Read the model definition and answer for the solid it produces. Units are mm, in the model's axes. A direction names the side the tool comes from. Round coordinates to 2 decimals unless told otherwise and drop trailing zeros. Write each loop counter-clockwise with the first axis right and the second up, starting at its lowest first coordinate (ties: lowest second). Pieces come first, ordered by that corner, then holes.
from build123d import *

# Parameters (mm, degrees)
BOSS_EXTRUDE1_DEPTH = 6.35
SKETCH2_R           = 5.08
BOSS_EXTRUDE2_DEPTH = 6.35
SKETCH3_R           = 5.08
BOSS_EXTRUDE3_DEPTH = 19.05
SKETCH4_R           = 3.81
CUT_EXTRUDE1_DEPTH  = 32.75
CUT_EXTRUDE2_DEPTH  = 15.24
CIRPATTERN1_COUNT   = 6


with BuildPart() as part:
    # Sketch1 → Boss-Extrude1 (new body)
    with BuildSketch(Plane.XY):
        Polygon((0, 8.248891971), (-7.14375, 4.124445986), (-7.14375, -4.124445986), (0, -8.248891971), (7.14375, -4.124445986), (7.14375, 4.124445986), align=None)
    extrude(amount=BOSS_EXTRUDE1_DEPTH)

    # Sketch2 → Boss-Extrude2 (add)
    with BuildSketch(Plane(origin=(0, 0, 0), x_dir=(-1, 0, 0), z_dir=(0, 0, -1))):
        Circle(SKETCH2_R)
    extrude(amount=BOSS_EXTRUDE2_DEPTH)

    # Sketch3 → Boss-Extrude3 (add)
    with BuildSketch(Plane.XY.offset(6.35)):
        Circle(SKETCH3_R)
    extrude(amount=BOSS_EXTRUDE3_DEPTH)

    # Sketch4 → Cut-Extrude1 (cut, through all)
    with BuildSketch(Plane.XY.offset(25.4)):
        Circle(SKETCH4_R)
    extrude(amount=-CUT_EXTRUDE1_DEPTH, mode=Mode.SUBTRACT)

    # Sketch5 → Cut-Extrude2 (cut)
    with BuildSketch(Plane.XY.offset(25.4)):
        Polygon((0, 4.810914796), (0.765045953, 4.810914796), (1.27, 5.114868927), (0, 5.114868927), (-1.27, 5.114868927), (-0.765045953, 4.810914796), align=None)
    cut_extrude2 = extrude(amount=-CUT_EXTRUDE2_DEPTH, mode=Mode.SUBTRACT)

    # CirPattern1: Cut-Extrude2 ×6 about axis
    cirpattern1_axis = Axis((0, 0, 0), (0, 0, 1))
    for i in range(1, CIRPATTERN1_COUNT):
        add(cut_extrude2.rotate(cirpattern1_axis, i * 360 / CIRPATTERN1_COUNT), mode=Mode.SUBTRACT)


solid = part.part
Q1. Determine the mould class of faces 1 (the cylindrical face through (-0.83, -3.72, 9.75)), 2 (the flat face through (3.522, -6.216, 3.131)), 3 (the flat face through (-3.522, 6.216, 3.131)) for opening direction X: pulls with the +X half, pulls with the -X half, needs draft (parallel to the pull), parting line crosses it, or undercut.
Verdict:
face 1: undercut
face 2: pulls with the +X half
face 3: pulls with the -X half
Q2. Straight lines are drawn through the part: probe 1 along Y at (x, z) = (0, 13); probe 2 along Y at (x, z) = (0, 8.5); probe 3 along Z at (x, y) = (4, 4.5). For each, find the intervals that lie inside material, in ascending order.
Verdict:
probe 1: y = -4.81 to -3.81, 3.81 to 4.81
probe 2: y = -5.08 to -3.81, 3.81 to 5.08
probe 3: z = 0 to 6.35
Q3. Section A-A (x = -2.25) is taken. Determine the outline of the cut face in (y, z), then the cut area to 3 significant figures.
Verdict:
outline: (-6.95, 0) - (-4.55, 0) - (-4.55, -6.35) - (-3.07, -6.35) - (-3.07, 25.4) - (-4.55, 25.4) - (-4.55, 6.35) - (-6.95, 6.35) - close; (3.07, -6.35) - (4.55, -6.35) - (4.55, 0) - (6.95, 0) - (6.95, 6.35) - (4.55, 6.35) - (4.55, 25.4) - (3.07, 25.4) - close
area: 124 mm2
Q4. Which of the six approach directions +Z, -Z, +X, -X, +Y, -Y give full straight-line access (tool end or side, diameter ignored) to faces 4 (the cylindrical face through (0.661, 5.037, -3.131)), 5 (the flat face through (-4.161, -2.415, 17.887)), 6 (the flat face through (-5, -2, 6.35))?
Verdict:
face 4: -Z
face 5: +Z, -X, -Y
face 6: +Z
Q5. Section C-C (z = 10.5) is taken. Determine the outline of the cut face in (x, y), then the cut area to 3 significant figures.
Verdict:
outline: (-4.82, -1.59) - (-4.55, -1.74) - (-3.78, -3.07) - (-3.79, -3.38) arc R5.08 ccw to (-1.04, -4.97) - (-0.77, -4.81) - (0.77, -4.81) - (1.04, -4.97) arc R5.08 ccw to (3.79, -3.38) - (3.78, -3.07) - (4.55, -1.74) - (4.82, -1.59) arc R5.08 ccw to (4.82, 1.59) - (4.55, 1.74) - (3.78, 3.07) - (3.79, 3.38) arc R5.08 ccw to (1.04, 4.97) - (0.77, 4.81) - (-0.77, 4.81) - (-1.04, 4.97) arc R5.08 ccw to (-3.79, 3.38) - (-3.78, 3.07) - (-4.55, 1.74) - (-4.82, 1.59) arc R5.08 ccw to start; hole circle Ø7.62 at (0, 0)
area: 32.8 mm2
Q6. Section D-D (y = -4.5) is taken. Determine the outline of the cut face in (x, z), then the cut area to 3 significant figures.
Verdict:
outline: (-6.49, 0) - (-2.36, 0) - (-2.36, -6.35) - (2.36, -6.35) - (2.36, 0) - (6.49, 0) - (6.49, 6.35) - (2.36, 6.35) - (2.36, 25.4) - (-2.36, 25.4) - (-2.36, 6.35) - (-6.49, 6.35) - close
area: 202 mm2
Q7. Section B-B (y = 0) is taken. Determine the outline of the cut face in (x, z), then the cut area to 3 significant figures.
Verdict:
outline: (-7.14, 0) - (-5.08, 0) - (-5.08, -6.35) - (-3.81, -6.35) - (-3.81, 25.4) - (-5.08, 25.4) - (-5.08, 6.35) - (-7.14, 6.35) - close; (3.81, -6.35) - (5.08, -6.35) - (5.08, 0) - (7.14, 0) - (7.14, 6.35) - (5.08, 6.35) - (5.08, 25.4) - (3.81, 25.4) - close
area: 107 mm2
Q8. Flat-ended cylindrical pins translate along their axes: pin 1 Ø3 at (x, z) = (-2, 11) entering from +Y; pin 2 Ø4 at (x, z) = (-4.5, 17.5) entering from -Y; pin 3 Ø1.5 at (x, y) = (1.5, 6.5) entering from -Z; pin 4 Ø6 at (x, y) = (0, 0) entering from -Z. Find the tip coordinate at first contact, or state that the pin passes through.
Verdict:
pin 1: stops at y = 5.02
pin 2: stops at y = -4.42
pin 3: stops at z = 0
pin 4: passes through
